```python
from build123d import *

# Parameters (mm, degrees)
SKETCH1_W           = 300
SKETCH1_H           = 120
BOSS_EXTRUDE1_DEPTH = 4
SKETCH2_W           = 300
SKETCH2_H           = 120
SKETCH2_W_2         = 292
SKETCH2_H_2         = 112
BOSS_EXTRUDE2_DEPTH = 140
FILLET1_R           = 5
BOSS_EXTRUDE3_DEPTH = 4
FILLET2_R           = 2
CUT_EXTRUDE1_REACH  = 312
SKETCH4_R           = 2.25
CUT_EXTRUDE2_REACH  = 132
SKETCH5_R           = 2.25


with BuildPart() as part:
    # Sketch1 → Boss-Extrude1 (new body)
    with BuildSketch(Plane(origin=(0, 0, 0), x_dir=(1, 0, 0), z_dir=(0, 1, 0))):
        Rectangle(SKETCH1_W, SKETCH1_H)
    extrude(amount=BOSS_EXTRUDE1_DEPTH)

    # Sketch2 → Boss-Extrude2 (add)
    with BuildSketch(Plane(origin=(0, 4, 0), x_dir=(1, 0, 0), z_dir=(0, 1, 0))):
        Rectangle(SKETCH2_W, SKETCH2_H)
        Rectangle(SKETCH2_W_2, SKETCH2_H_2, mode=Mode.SUBTRACT)
    extrude(amount=BOSS_EXTRUDE2_DEPTH)

    # Fillet1
    fillet1_edges = [part.edges().sort_by_distance(p)[0] for p in [
        (-146, 74, 56),
        (146, 74, 56),
        (146, 74, -56),
        (-146, 74, -56),
        (-150, 72, -60),
        (150, 72, -60),
        (150, 72, 60),
        (-150, 72, 60),
    ]]
    fillet(fillet1_edges, radius=FILLET1_R)

    # Sketch3 → Boss-Extrude3 (add)
    with BuildSketch(Plane(origin=(0, 144, 0), x_dir=(1, 0, 0), z_dir=(0, 1, 0))):
        with BuildLine():
            Line((-141, 70), (141, 70))
            ThreePointArc((141, 70), (154.435028843, 64.435028843), (160, 51))
            Line((160, 51), (160, -51))
            ThreePointArc((160, -51), (154.435028843, -64.435028843), (141, -70))
            Line((141, -70), (-141, -70))
            ThreePointArc((-141, -70), (-154.435028843, -64.435028843), (-160, -51))
            Line((-160, -51), (-160, 51))
            ThreePointArc((-160, 51), (-154.435028843, 64.435028843), (-141, 70))
        make_face()
        with BuildLine():
            Line((-141, 56), (141, 56))
            ThreePointArc((141, 56), (144.535533906, 54.535533906), (146, 51))
            Line((146, 51), (146, -51))
            ThreePointArc((146, -51), (144.535533906, -54.535533906), (141, -56))
            Line((141, -56), (-141, -56))
            ThreePointArc((-141, -56), (-144.535533906, -54.535533906), (-146, -51))
            Line((-146, -51), (-146, 51))
            ThreePointArc((-146, 51), (-144.535533906, 54.535533906), (-141, 56))
        make_face(mode=Mode.SUBTRACT)
    extrude(amount=BOSS_EXTRUDE3_DEPTH)

    # Fillet2
    fillet2_edges = [part.edges().sort_by_distance(p)[0] for p in [
        (0, 144, 60),
        (-150, 144, 0),
        (150, 144, 0),
        (0, 144, -60),
        (-148.535533906, 144, -58.535533906),
        (148.535533906, 144, -58.535533906),
        (148.535533906, 144, 58.535533906),
        (-148.535533906, 144, 58.535533906),
    ]]
    fillet(fillet2_edges, radius=FILLET2_R)

    # Sketch4 → Cut-Extrude1 (cut, up to next)
    with BuildSketch(Plane(origin=(150, 0, 0), x_dir=(0, 0, -1), z_dir=(1, 0, 0)), mode=Mode.PRIVATE) as cut_extrude1_sk1:
        with Locations((-15, 79)):
            Circle(SKETCH4_R)
    cut_extrude1_tool1 = extrude(cut_extrude1_sk1.sketch, amount=-CUT_EXTRUDE1_REACH, mode=Mode.PRIVATE) & part.part
    add(cut_extrude1_tool1.solids().sort_by_distance((150, 79, 15))[0], mode=Mode.SUBTRACT)
    # Sketch4 → Cut-Extrude1 (cut, up to next)
    with BuildSketch(Plane(origin=(150, 0, 0), x_dir=(0, 0, -1), z_dir=(1, 0, 0)), mode=Mode.PRIVATE) as cut_extrude1_sk2:
        with Locations((15, 79)):
            Circle(SKETCH4_R)
    cut_extrude1_tool2 = extrude(cut_extrude1_sk2.sketch, amount=-CUT_EXTRUDE1_REACH, mode=Mode.PRIVATE) & part.part
    add(cut_extrude1_tool2.solids().sort_by_distance((150, 79, -15))[0], mode=Mode.SUBTRACT)
    # Sketch4 → Cut-Extrude1 (cut, up to next)
    with BuildSketch(Plane(origin=(150, 0, 0), x_dir=(0, 0, -1), z_dir=(1, 0, 0)), mode=Mode.PRIVATE) as cut_extrude1_sk3:
        with Locations((15, 40)):
            Circle(SKETCH4_R)
    cut_extrude1_tool3 = extrude(cut_extrude1_sk3.sketch, amount=-CUT_EXTRUDE1_REACH, mode=Mode.PRIVATE) & part.part
    add(cut_extrude1_tool3.solids().sort_by_distance((150, 40, -15))[0], mode=Mode.SUBTRACT)
    # Sketch4 → Cut-Extrude1 (cut, up to next)
    with BuildSketch(Plane(origin=(150, 0, 0), x_dir=(0, 0, -1), z_dir=(1, 0, 0)), mode=Mode.PRIVATE) as cut_extrude1_sk4:
        with Locations((-15, 40)):
            Circle(SKETCH4_R)
    cut_extrude1_tool4 = extrude(cut_extrude1_sk4.sketch, amount=-CUT_EXTRUDE1_REACH, mode=Mode.PRIVATE) & part.part
    add(cut_extrude1_tool4.solids().sort_by_distance((150, 40, 15))[0], mode=Mode.SUBTRACT)

    # Sketch5 → Cut-Extrude2 (cut, up to next)
    with BuildSketch(Plane.XY.offset(60), mode=Mode.PRIVATE) as cut_extrude2_sk1:
        with Locations((15, 79)):
            Circle(SKETCH5_R)
    cut_extrude2_tool1 = extrude(cut_extrude2_sk1.sketch, amount=-CUT_EXTRUDE2_REACH, mode=Mode.PRIVATE) & part.part
    add(cut_extrude2_tool1.solids().sort_by_distance((15, 79, 60))[0], mode=Mode.SUBTRACT)
    # Sketch5 → Cut-Extrude2 (cut, up to next)
    with BuildSketch(Plane.XY.offset(60), mode=Mode.PRIVATE) as cut_extrude2_sk2:
        with Locations((-15, 79)):
            Circle(SKETCH5_R)
    cut_extrude2_tool2 = extrude(cut_extrude2_sk2.sketch, amount=-CUT_EXTRUDE2_REACH, mode=Mode.PRIVATE) & part.part
    add(cut_extrude2_tool2.solids().sort_by_distance((-15, 79, 60))[0], mode=Mode.SUBTRACT)
    # Sketch5 → Cut-Extrude2 (cut, up to next)
    with BuildSketch(Plane.XY.offset(60), mode=Mode.PRIVATE) as cut_extrude2_sk3:
        with Locations((-15, 40)):
            Circle(SKETCH5_R)
    cut_extrude2_tool3 = extrude(cut_extrude2_sk3.sketch, amount=-CUT_EXTRUDE2_REACH, mode=Mode.PRIVATE) & part.part
    add(cut_extrude2_tool3.solids().sort_by_distance((-15, 40, 60))[0], mode=Mode.SUBTRACT)
    # Sketch5 → Cut-Extrude2 (cut, up to next)
    with BuildSketch(Plane.XY.offset(60), mode=Mode.PRIVATE) as cut_extrude2_sk4:
        with Locations((15, 40)):
            Circle(SKETCH5_R)
    cut_extrude2_tool4 = extrude(cut_extrude2_sk4.sketch, amount=-CUT_EXTRUDE2_REACH, mode=Mode.PRIVATE) & part.part
    add(cut_extrude2_tool4.solids().sort_by_distance((15, 40, 60))[0], mode=Mode.SUBTRACT)


solid = part.part
```
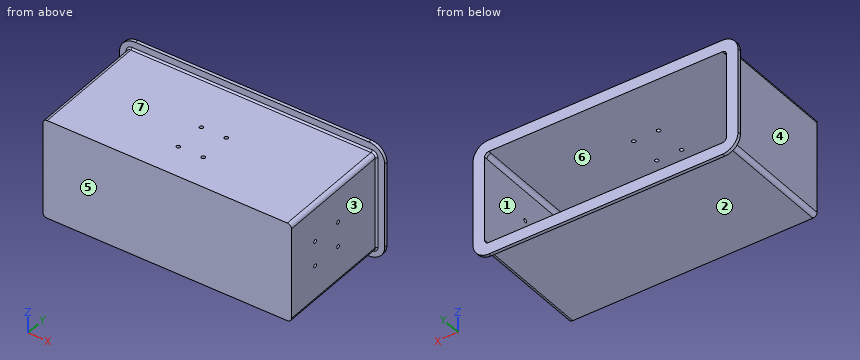
Can you work these out from the model? Positions are in its coordinate system, mm. Face numbers are marked on the shaded views. A direction names the side the tool comes from. Round coordinates to 2 decimals unless told otherwise and drop trailing zeros. Loops run counter-clockwise (first coordinate to the right, second up) from the corner with the lowest first, then second, coordinate; pieces in that order, holes last. Notation, with made-up numbers: M 8.25,43 L 64.25,43 A13 ccw 64.25,67 Z; hole C 78.25,-11.75 d9. An arc over 180 degrees is marked long. Answer in a Markdown table with one row per item.
1. I'm going to push flat-ended pins straight in: pin 1 Ø1 at (y, z) = (97.5, -2.5) entering from +X; pin 2 Ø1.5 at (x, y) = (-53, 91) entering from -Z; pin 3 Ø10 at (y, z) = (44.5, 43.5) entering from -X. Where does each tip first touch, or does it pass through?
Established:
| item | result |
|---|---|
| pin 1 | x = 150 |
| pin 2 | z = -60 |
| pin 3 | x = -150 |
2. Thinking about a two-plate mould opening in X: for the marked faces 1, 2, 3 and 4, which applies, pulls with the +X half, pulls with the -X half, needs draft (parallel to the pull), parting line crosses it, or undercut?
Established:
| item | result |
|---|---|
| face 1 | undercut |
| face 2 | needs draft |
| face 3 | pulls with the +X half |
| face 4 | pulls with the -X half |
3. If we section it at C-C, the plane z = 46: Please give me the cut outline in (x, y).
Established:
| item | result |
|---|---|
| outline | M -160,144 L -152,144 A2 cw -150,142 L -150,0 L 150,0 L 150,142 A2 cw 152,144 L 160,144 L 160,148 L 146,148 L 146,4 L -146,4 L -146,148 L -160,148 Z |
4. Please list where these lines run through material, in increasing order: line 1 (Y direction, x = 15, z = 58); line 2 (X direction, y = 125, z = 1.5); line 3 (Z direction, x = -121, y = 106.5). Write a range as from..to.
Established:
| item | result |
|---|---|
| line 1 | 0..37.75, 42.25..76.75, 81.25..148 |
| line 2 | -150..-146, 146..150 |
| line 3 | -60..-56, 56..60 |
5. On a 3-axis mill with a long thin cutter (end or side, diameter ignored), from which of +Z, -Z, +X, -X, +Y, -Y can I reach the whole of each face in a straight line? I mean the marked faces 5, 6 and 7. Say none if no direction works.
Established:
| item | result |
|---|---|
| face 5 | +Z, -Z, +X, -X, -Y |
| face 6 | +Y |
| face 7 | +Z, +X, -X, -Y |
6. If we section it at B-B, the plane x = 59: Please give me the cut outline in (y, z), plus the area to 3 significant figures.
Established:
| item | result |
|---|---|
| outline | M 0,-60 L 142,-60 A2 cw 144,-62 L 144,-70 L 148,-70 L 148,-56 L 4,-56 L 4,56 L 148,56 L 148,70 L 144,70 L 144,62 A2 cw 142,60 L 0,60 Z |
| area | 1,710 mm² |
7. If we section it at A-A, the plane y = 117: Please give me the cut outline in (x, z), plus the area to 3 significant figures.
Established:
| item | result |
|---|---|
| outline | M -150,-55 A5 ccw -145,-60 L 145,-60 A5 ccw 150,-55 L 150,55 A5 ccw 145,60 L -145,60 A5 ccw -150,55 Z; hole M -146,-51 A5 ccw -141,-56 L 141,-56 A5 ccw 146,-51 L 146,51 A5 ccw 141,56 L -141,56 A5 ccw -146,51 Z |
| area | 3,300 mm² |
